from build123d import *

# Parameters (mm, degrees)
RESSALTO_EXTRUS_O1_DEPTH      = 5
ESBO_O4_W                     = 92.887769858
ESBO_O4_H                     = 14.984754445
CORTE_EXTRUS_O1_DEPTH         = 3
RESSALTO_EXTRUS_O12_OUTLINE_W = 22.942167962
RESSALTO_EXTRUS_O12_OUTLINE_H = 18.018363384
RESSALTO_EXTRUS_O12_DEPTH     = 2.068801543
ESBO_O10_W                    = 24.255846062
ESBO_O10_H                    = 9.941166005
RESSALTO_EXTRUS_O2_DEPTH      = 9
ESBO_O12_W                    = 24.5665075
ESBO_O12_H                    = 9.941166005
RESSALTO_EXTRUS_O3_DEPTH      = 9
ESBO_O13_W                    = 22.942167962
ESBO_O13_H                    = 33.982493236
RESSALTO_EXTRUS_O4_DEPTH      = 3
ESBO_O14_W                    = 6.782835172
ESBO_O14_H                    = 7.872436605
ESBO_O14_W_2                  = 6.782835171
ESBO_O14_H_2                  = 7.872436606
CORTE_EXTRUS_O4_DEPTH         = 3
ESBO_O15_W                    = 19.105678415
ESBO_O15_H                    = 14.135095414
RESSALTO_EXTRUS_O5_DEPTH      = 1
ESBO_O18_W                    = 6.523890191
ESBO_O18_H                    = 6.679220909
RESSALTO_EXTRUS_O9_DEPTH      = 10
ESBO_O19_W                    = 7.766535942
ESBO_O19_H                    = 7.300543785
RESSALTO_EXTRUS_O10_DEPTH     = 15
ESBO_O21_W                    = 13.689709829
ESBO_O21_H                    = 4.124463858
RESSALTO_EXTRUS_O13_DEPTH     = 11
ESBO_O22_W                    = 3.40794345
ESBO_O22_H                    = 8.387858817
ESBO_O22_W_2                  = 3.845821911
RESSALTO_EXTRUS_O14_DEPTH     = 6
ESBO_O23_R                    = 1.902232627
ESBO_O23_R_2                  = 1.546559196
ESBO_O23_W                    = 8.387858817
ESBO_O23_H                    = 4.038598689
RESSALTO_EXTRUS_O15_DEPTH     = 8


# Read off the part's stored shape, not the designer's step: Ressalto-extrusão12
with BuildPart() as part:
    # Esboço2 → Ressalto-extrusão1 (new body)
    with BuildSketch(Plane.XY):
        Polygon((-71.39802883, 58.87134079), (-32.546471332, 58.87134079), (-32.546471332, 79.355053275), (-71.39802883, 79.355053275), (-71.39802883, 99.40294209), (28.994123383, 99.40294209), (28.994123383, 79.355053275), (-9.60430337, 79.355053275), (-9.60430337, 58.87134079), (28.994123383, 58.87134079), (28.994123383, -18.483753656), (-71.39802883, -18.483753656), align=None)
    extrude(amount=RESSALTO_EXTRUS_O1_DEPTH)

    # Esboço4 → Corte-extrusão1 (cut)
    with BuildSketch(Plane.XY.offset(5)):
        with Locations((-20.735960567, 91.910564867)):
            Rectangle(ESBO_O4_W, ESBO_O4_H)
    extrude(amount=-CORTE_EXTRUS_O1_DEPTH, mode=Mode.SUBTRACT)

    # Ressalto-extrusão12 outline → Ressalto-extrusão12 (add)
    with BuildSketch(Plane.XY.offset(5)):
        with Locations((-21.075387351, 3.180221698)):
            Rectangle(RESSALTO_EXTRUS_O12_OUTLINE_W, RESSALTO_EXTRUS_O12_OUTLINE_H)
    extrude(amount=RESSALTO_EXTRUS_O12_DEPTH)

    # Esboço10 → Ressalto-extrusão2 (add)
    with BuildSketch(Plane.XY.offset(5)):
        with Locations((-59.270105799, 7.840143264)):
            Rectangle(ESBO_O10_W, ESBO_O10_H)
    extrude(amount=RESSALTO_EXTRUS_O2_DEPTH)

    # Esboço12 → Ressalto-extrusão3 (add)
    with BuildSketch(Plane.XY.offset(5)):
        with Locations((16.710869633, 7.840143264)):
            Rectangle(ESBO_O12_W, ESBO_O12_H)
    extrude(amount=RESSALTO_EXTRUS_O3_DEPTH)

    # Esboço13 → Ressalto-extrusão4 (add)
    with BuildSketch(Plane.XY.offset(5)):
        with Locations((-21.075387351, 36.942158983)):
            Rectangle(ESBO_O13_W, ESBO_O13_H)
    extrude(amount=RESSALTO_EXTRUS_O4_DEPTH)

    # Esboço14 → Corte-extrusão4 (cut)
    with BuildSketch(Plane.XY.offset(2)):
        with Locations((-49.698600708, 93.563993113)):
            Rectangle(ESBO_O14_W, ESBO_O14_H)
        with Locations((-14.471948292, 93.556871263)):
            Rectangle(ESBO_O14_W, ESBO_O14_H)
        with Locations((-38.766760461, 93.495131296)):
            Rectangle(ESBO_O14_W_2, ESBO_O14_H_2)
        with Locations((-27.731681244, 93.42626948)):
            Rectangle(ESBO_O14_W, ESBO_O14_H)
        with Locations((-59.769614495, 93.632854929)):
            Rectangle(ESBO_O14_W_2, ESBO_O14_H_2)
        with Locations((-3.484568548, 93.465026179)):
            Rectangle(ESBO_O14_W, ESBO_O14_H_2)
        with Locations((7.375442348, 93.465026179)):
            Rectangle(ESBO_O14_W, ESBO_O14_H_2)
        with Locations((18.235453244, 93.696013601)):
            Rectangle(ESBO_O14_W, ESBO_O14_H_2)
    extrude(amount=-CORTE_EXTRUS_O4_DEPTH, mode=Mode.SUBTRACT)

    # Esboço15 → Ressalto-extrusão5 (add)
    with BuildSketch(Plane.XY.offset(8)):
        with Locations((-20.813625927, 29.974770696)):
            Rectangle(ESBO_O15_W, ESBO_O15_H)
    extrude(amount=RESSALTO_EXTRUS_O5_DEPTH)

    # Esboço18 → Ressalto-extrusão9 (add)
    with BuildSketch(Plane(origin=(28.994123383, 0, 0), x_dir=(0, 0, -1), z_dir=(1, 0, 0))):
        with Locations((-9.174630064, 7.917808623)):
            Rectangle(ESBO_O18_W, ESBO_O18_H)
    extrude(amount=RESSALTO_EXTRUS_O9_DEPTH)

    # Esboço19 → Ressalto-extrusão10 (add)
    with BuildSketch(Plane.ZY.offset(71.39802883)):
        with Locations((9.185815902, 7.917808623)):
            Rectangle(ESBO_O19_W, ESBO_O19_H)
    extrude(amount=RESSALTO_EXTRUS_O10_DEPTH)

    # Esboço21 → Ressalto-extrusão13 (add)
    with BuildSketch(Plane.XY.offset(7.068801543)):
        with Locations((-21.156578629, -2.799751995)):
            Rectangle(ESBO_O21_W, ESBO_O21_H)
    extrude(amount=RESSALTO_EXTRUS_O13_DEPTH)

    # Esboço22 → Ressalto-extrusão14 (add)
    with BuildSketch(Plane.XY.offset(7.068801543)):
        with Locations((-30.842499607, 6.752828232)):
            Rectangle(ESBO_O22_W, ESBO_O22_H)
        with Locations((-11.527214326, 6.752828232)):
            Rectangle(ESBO_O22_W_2, ESBO_O22_H)
    extrude(amount=RESSALTO_EXTRUS_O14_DEPTH)

    # Esboço23 → Ressalto-extrusão15 (add)
    with BuildSketch(Plane.XY.offset(5)):
        with Locations((-15.988396591, 6.837106018)):
            Circle(ESBO_O23_R)
        with Locations((-25.960235387, 5.97818713)):
            Circle(ESBO_O23_R_2)
        with Locations((-22.92529913, 10.170104046)):
            Rectangle(ESBO_O23_W, ESBO_O23_H)
    extrude(amount=RESSALTO_EXTRUS_O15_DEPTH)


solid = part.part
Work out the finished part from the listing and answer in its coordinate system (mm). A direction names the side the tool comes from. Coordinates: 2 decimals unless noted, no trailing zeros. Order: outer loops, then holes, each group sorted by start corner. A loop starts at its lowest first (then second) coordinate and runs counter-clockwise, first axis right, second up. Notation, with made-up numbers: (-34, 10.25) - (6, 10.25) arc R11 ccw to (6, 16.25) - close; hole circle Ø10 at (31, -19). An arc over 180 degrees is marked (long way). Put each result on its own line as item: value. Start each with the question number.
1) Find the intervals of material crossed by line 1 (Y direction, x = 1.5, z = 1.75); line 2 (Z direction, x = 25.5, y = 93); line 3 (X direction, y = 51.5, z = 6), in increasing order. Write a range as from..to.
2) For faces 1 (the flat face through (-79, 8, 13.069)), 2 (the flat face through (4.428, 8, 9)), 3 (the flat face through (-21, 90, 2)), 4 (the flat face through (10, 79.355, 2)), 5 (the flat face through (34, 11.257, 9)), determine the directions among +Z, -Z, +X, -X, +Y, -Y from which every point of the face is accessible in a straight line to the end or side of a thin tool.
3) Find section D-D (z = 16.5). Give the vertices of the cut face in (x, y).
4) Find section C-C (x = 27.5). Give the vertices of the cut face in (y, z), plus the area to 3 significant figures.
5) For a pull along X with two mould halves and no side action, classify faces 6 (the flat face through (-14.312, -3, 12)), 7 (the flat face through (-23, 10, 13)), 8 (the flat face through (-12, 2.559, 10)) as released by +X, released by -X, zero draft, split by the parting line, or undercut.
6) Find section A-A (x = 12.5). Give the vertices of the cut face in (y, z).
7) Flat-ended cylindrical pins translate along their axes: pin 1 (2.5 mm diameter, centred on x = -30.5, y = 7, fed in from +Z); pin 2 (6 mm diameter, centred on x = -79, z = 8.5, fed in from -Y); pin 3 (7 mm diameter, centred on x = 17.5, z = 10, fed in from -Y); pin 4 (5.5 mm diameter, centred on x = -24.5, y = 0.5, fed in from +Z). Find the tip coordinate at first contact, or state that the pin passes through.
8) Find section B-B (y = 45.5). Give the vertices of the cut face in (x, z).
Results list:
1. line 1: y = -18.48..58.87, 79.36..99.4
1. line 2: z = 0..2
1. line 3: x = -32.55..-9.6
2. face 1: +Z, -X, +Y, -Y
2. face 2: +Z, +Y, -Y
2. face 3: +Z, +Y
2. face 4: +Z, -Z, +X
2. face 5: +Z, -Z, +X, +Y
3. outline: (-28, -4.86) - (-14.31, -4.86) - (-14.31, -0.74) - (-28, -0.74) - close
4. outline: (-18.48, 0) - (58.87, 0) - (58.87, 5) - (12.81, 5) - (12.81, 14) - (2.87, 14) - (2.87, 5) - (-18.48, 5) - close; (79.36, 0) - (99.4, 0) - (99.4, 5) - (79.36, 5) - close
4. area: 576 mm^2
5. face 6: released by +X
5. face 7: undercut
5. face 8: zero draft
6. outline: (-18.48, 0) - (58.87, 0) - (58.87, 5) - (12.81, 5) - (12.81, 14) - (2.87, 14) - (2.87, 5) - (-18.48, 5) - close; (79.36, 0) - (99.4, 0) - (99.4, 2) - (84.42, 2) - (84.42, 5) - (79.36, 5) - close
7. pin 1: stops at z = 13.07
7. pin 2: stops at y = 4.27
7. pin 3: stops at y = 2.87
7. pin 4: stops at z = 18.07
8. outline: (-71.4, 0) - (28.99, 0) - (28.99, 5) - (-9.6, 5) - (-9.6, 8) - (-32.55, 8) - (-32.55, 5) - (-71.4, 5) - close
